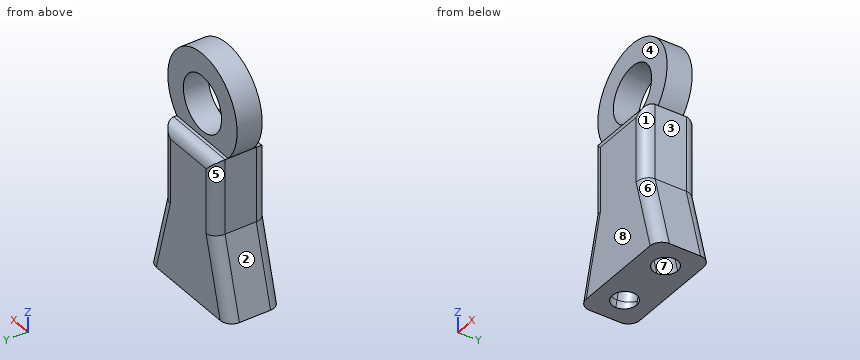
```python
from build123d import *

# Parameters (mm, degrees)
F0_R     = 8.485
F0_R_2   = 4.675
F1_DEPTH = 2.125
F2_W     = 12.5812107759
F2_H     = 12.7
F3_DEPTH = 4.539996
F5_DEPTH = 2.0625
F6_R     = 2.06249
F7_R     = 1.905


# Not quite as in the source:
# - a fillet or chamfer is up to 0.001 mm smaller than in the source, because OpenCascade refuses the exact size


with BuildPart() as f1:
    # F0 (on Front) → F1 (new body, symmetric)
    with BuildSketch(Plane.XZ):
        Circle(F0_R)
        Circle(F0_R_2, mode=Mode.SUBTRACT)
    extrude(amount=F1_DEPTH, both=True)

    # F2 (on Front) → F3 (join, symmetric)
    with BuildSketch(Plane.XZ):
        Polygon((-6.2906053879, -18.3941644561), (-9.7885362858, -31.4486202883), (9.7885362858, -31.4486202883), (6.2906053879, -18.3941644561), align=None)
        with Locations((0, -12.0441644561)):
            Rectangle(F2_W, F2_H)
    extrude(amount=F3_DEPTH, both=True)

    # F4 (on Front) → F5 (cut, symmetric)
    with BuildSketch(Plane.XZ):
        Polygon((4.22592549, -20.5024805709), (0.2414814566, -21.5701091319), (2.8884205433, -31.4486202883), (7.1589347875, -31.4486202883), align=None)
        Polygon((-0.2414814566, -21.5701091319), (-4.22592549, -20.5024805709), (-6.8555269883, -30.3162869659), (-7.1589347875, -31.4486202883), (-2.8884205433, -31.4486202883), align=None)
    extrude(amount=F5_DEPTH, both=True, mode=Mode.SUBTRACT)

    # F6 (radius 2.0625 in the source; OpenCascade refuses exactly that, so slightly less here)
    f6_edges = [f1.edges().sort_by_distance(p)[0] for p in [
        (-5.69243, -2.0625, -25.97555),
        (1.564951, -2.0625, -26.509365),
        (5.69243, -2.0625, -25.97555),
        (-1.564951, -2.0625, -26.509365),
        (5.69243, 2.0625, -25.97555),
        (-1.564951, 2.0625, -26.509365),
        (-5.69243, 2.0625, -25.97555),
        (1.564951, 2.0625, -26.509365),
    ]]
    fillet(f6_edges, radius=F6_R)

    # F7
    f7_edges = [f1.edges().sort_by_distance(p)[0] for p in [
        (-8.039571, -4.539996, -24.921392),
        (-6.290605, -4.539996, -12.044164),
        (-6.290605, 4.539996, -12.044164),
        (-8.039571, 4.539996, -24.921392),
        (8.039571, -4.539996, -24.921392),
        (6.290605, -4.539996, -12.044164),
        (8.039571, 4.539996, -24.921392),
        (6.290605, 4.539996, -12.044164),
        (0, 4.539996, -5.694164),
        (0, -4.539996, -5.694164),
    ]]
    fillet(f7_edges, radius=F7_R)


solid = f1.part
```
The model under review builds one solid part; all positions refer to its coordinate system, in mm. Face numbers are marked on the shaded views. A direction names the side the tool comes from. Round coordinates to 2 decimals unless told otherwise and drop trailing zeros. Loops run counter-clockwise (first coordinate to the right, second up) from the corner with the lowest first, then second, coordinate; pieces in that order, holes last. Notation, with made-up numbers: (-18, 24) - (-8, 24) arc R35 ccw to (-8, 56) - close; hole circle Ø8 at (69, 83). An arc over 180 degrees is marked (long way). Use a Markdown table: item, result. Add a question column.
Q1. The part is to be moulded in two halves that separate along X. For the marked faces 6, 7 and 8, say which applies: pulls with the +X half, pulls with the -X half, needs draft (parallel to the pull), parting line crosses it, or undercut.
Q2. Add section B-B (x = 1). State how many separate pieces and enclosed holes the cut face has, plus the area to 3 significant figures.
Q3. Add section C-C (y = 3). State the section outline as (x, z) points.
Q4. Add section A-A (z = 0). State the section outline as (x, y) points (3 decimals), plus the area to 3 significant figures.
Q5. For probe 1 along X at (y, z) = (-1.75, -25); probe 2 along Y at (x, z) = (6.25, -2) (3 decimals); probe 3 along Y at (x, z) = (-4, -28), list the stretches that pass through material, from the lowest coordinate up.
Q6. Machinability: for the marked faces 1, 2, 3, 4 and 5, which of the approach directions +Z, -Z, +X, -X, +Y, -Y give a long, thin tool a straight path to every point of the face, cutting with its end or side? Answer none if there is none.
Q7. Insertion check: pin 1 Ø4.5 at (x, z) = (2.5, 2.5) entering from +Y (3 decimals); pin 2 Ø4 at (y, z) = (3.5, -20.5) entering from +X; pin 3 Ø2 at (x, y) = (5, -1) entering from +Z; pin 4 Ø3 at (x, z) = (2.5, -0.5) entering from +Y. Each pin has a flat end and moves straight along its axis. Give the tip position at first contact, or say it passes through.
Worked answers:
| question | item | result |
|---|---|---|
| 1 | face 6 | pulls with the +X half |
| 1 | face 7 | undercut |
| 1 | face 8 | needs draft |
| 2 | separate pieces | 2 |
| 2 | enclosed holes | 1 |
| 2 | area | 247 mm² |
| 3 | outline | (-9.75, -31.45) - (9.75, -31.45) - (6.26, -18.4) - (6.26, -5.73) - (-6.26, -5.73) - (-6.26, -18.4) - close |
| 4 | outline | (-8.485, -2.125) - (-4.675, -2.125) - (-4.675, 2.125) - (-8.485, 2.125) - close; (4.675, -2.125) - (8.485, -2.125) - (8.485, 2.125) - (4.675, 2.125) - close |
| 4 | area | 32.4 mm² |
| 5 | probe 1 | -8.06 to -4.43, -2.17 to 2.17, 4.43 to 8.06 |
| 5 | probe 2 | -2.125 to 2.125 |
| 5 | probe 3 | -4.54 to -2.06, 2.06 to 4.54 |
| 6 | face 1 | +Z, +X, -Y |
| 6 | face 2 | -X, +Y, -Y |
| 6 | face 3 | +X, +Y, -Y |
| 6 | face 4 | +Z, +X, -X, -Y |
| 6 | face 5 | +Z, -X, +Y |
| 7 | pin 1 | y = 2.125 |
| 7 | pin 2 | x = 7.35 |
| 7 | pin 3 | z = 7.48 |
| 7 | pin 4 | through |
